Can you work these out from the model? Positions are in its coordinate system, mm. A direction names the side the tool comes from. Give positions to 0.01 mm unless a question says otherwise; leave off trailing zeros. Loops run counter-clockwise (first coordinate to the right, second up) from the corner with the lowest first, then second, coordinate; pieces in that order, holes last. Notation, with made-up numbers: M -26.5,15 L -5.5,15 A19 cw -5.5,33 Z; hole C -30,10.25 d4. An arc over 180 degrees is marked long. Answer as a JSON object with one key per item and string values.
```python
from build123d import *

# Parameters (mm, degrees)
EXTRUDE_1_DEPTH = 10
FILLET_1_R      = 3
FILLET_2_R      = 10
M4X0_71_D       = 3.3
FILLET_3_R      = 2


with BuildPart() as part:
    # Эскиз1 → Бобышка-Вытянуть1 (new body)
    with BuildSketch(Plane(origin=(0, 0, 0), x_dir=(1, 0, 0), z_dir=(0, 1, 0))):
        Polygon((0, 11), (-40, 3), (-40, 0), (-50, 0), (-50, 21), (50, 21), (50, 0), (40, 0), (40, 3), align=None)
    extrude(amount=EXTRUDE_1_DEPTH)

    # Скругление1
    fillet_1_edges = [part.edges().sort_by_distance(p)[0] for p in [
        (-40, 5, -3),
        (40, 5, -3),
    ]]
    fillet(fillet_1_edges, radius=FILLET_1_R)

    # Скругление2
    fillet_2_edges = [part.edges().sort_by_distance(p)[0] for p in [
        (0, 5, -11),
    ]]
    fillet(fillet_2_edges, radius=FILLET_2_R)

    # Отверстие обработанное метчиком M4x0.71 (through all)
    with Locations(Plane.XY):
        with Locations((-45, 5), (45, 5)):
            Hole(M4X0_71_D / 2)

    # Скругление3
    fillet_3_edges = [part.edges().sort_by_distance(p)[0] for p in [
        (40, 5, 0),
        (50, 5, 0),
        (50, 5, -21),
        (-50, 5, -21),
        (-50, 5, 0),
        (-40, 5, 0),
    ]]
    fillet(fillet_3_edges, radius=FILLET_3_R)


solid = part.part
```
1) For faces 1 (the flat face through (20, 5, -7)), 2 (the cylindrical face through (-49.4, 5.07, -0.57)), which set-ups out of +Z, -Z, +X, -X, +Y, -Y let a thin tool reach every point of the face, with its end or its side?
Answer list:
{"face 1": "+Z, +Y, -Y", "face 2": "+Z, -X, +Y, -Y"}
2) Suppose I cut it at B-B, the plane z = -13.25. Write out the boundary of the cut face in (x, y), and give its area (3 significant figures).
Answer list:
{"outline": "M -50,0 L 50,0 L 50,10 L -50,10 Z; hole C -45,5 d3.3; hole C 45,5 d3.3", "area": "983 mm^2"}
3) Suppose I cut it at C-C, the plane y = 5. Give the number of separate pieces and of enclosed holes in the cut face, and give its area (3 significant figures).
Answer list:
{"separate pieces": "3", "enclosed holes": "0", "area": "1,400 mm^2"}
4) Please list where these lines run through material, in increasing order: line 1 along X through (y, z) = (4.75, -12); line 2 along Y through (x, z) = (-45, -13.25); line 3 along X through (y, z) = (6.5, -15.5). Write a range as from..to.
Answer list:
{"line 1": "-50..-46.63, -43.37..43.37, 46.63..50", "line 2": "0..3.35, 6.65..10", "line 3": "-50..-45.69, -44.31..44.31, 45.69..50"}
5) If we mould it in two halves opening along Y, with no side actions, what happens to faces 3 (the flat face through (1, 10, -13)), 4 (the flat face through (-20, 5, -7)), 5 (the cylindrical face through (-43.35, 5.07, -10.65)), 6 (the cylindrical face through (46.65, 5.07, -10.65))? For each: +Y half, -Y half, draft (parallel to the pull), parting line (faces both ways), or undercut.
Answer list:
{"face 3": "+Y half", "face 4": "draft", "face 5": "undercut", "face 6": "undercut"}
6) Suppose I cut it at D-D, the plane x = -12.5. Write out the boundary of the cut face in (y, z), and give its area (3 significant figures).
Answer list:
{"outline": "M 0,-21 L 10,-21 L 10,-8.5 L 0,-8.5 Z", "area": "125 mm^2"}
7) Suppose I cut it at A-A, the plane x = -45. Write out the boundary of the cut face in (y, z).
Answer list:
{"outline": "M 0,-21 L 3.35,-21 L 3.35,0 L 0,0 Z; M 6.65,-21 L 10,-21 L 10,0 L 6.65,0 Z"}
